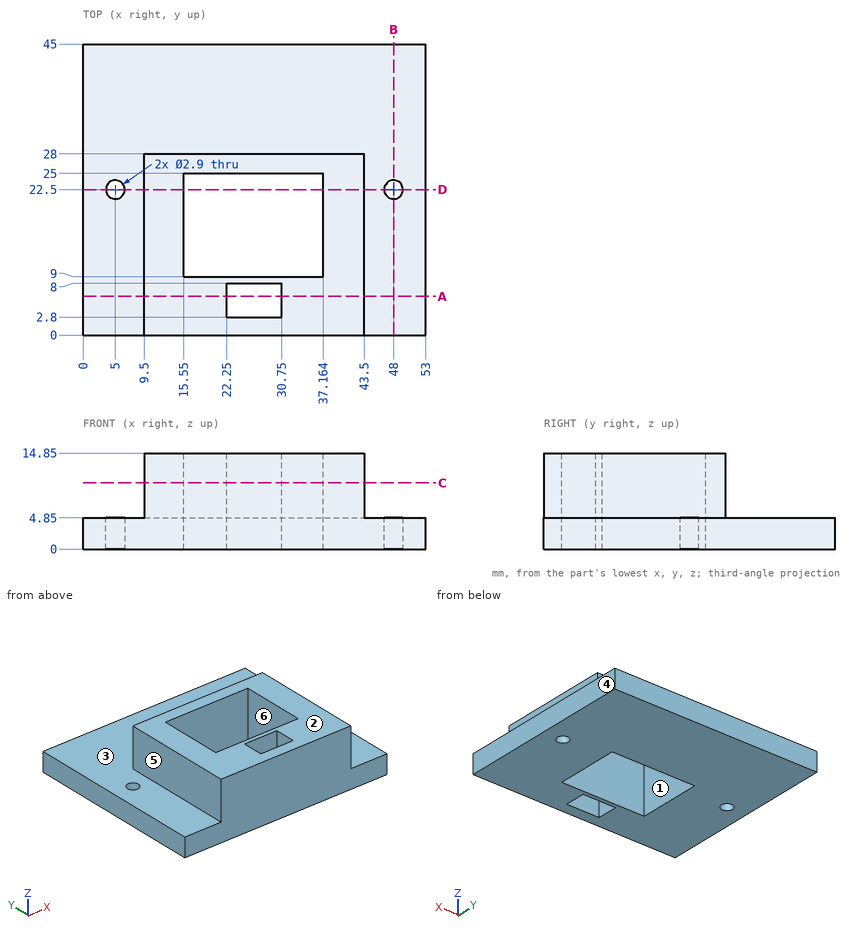
Design review of the part shown in the three views and the two pictorial views. Dimensions are in mm from the part's minimum x, y and z. A direction names the side the tool comes from. Round coordinates to 2 decimals unless told otherwise and drop trailing zeros. Loops run counter-clockwise (first coordinate to the right, second up) from the corner with the lowest first, then second, coordinate; pieces in that order, holes last. Notation, with made-up numbers: (40.25, 77) -> (80.25, 77) arc R19 ccw to (80.25, 83) -> close; hole circle Ø2 at (-2.75, 31.25). An arc over 180 degrees is marked (long way). Return JSON: item names as keys, results as strings.
(1) Add section C-C on z = 10.25. Write out the cut boundary in (x, y), plus the area to 3 significant figures.
Solved:
{"outline": "(9.5, 0) -> (43.5, 0) -> (43.5, 28) -> (9.5, 28) -> close; hole (15.55, 9) -> (37.16, 9) -> (37.16, 25) -> (15.55, 25) -> close; hole (22.25, 2.8) -> (30.75, 2.8) -> (30.75, 8) -> (22.25, 8) -> close", "area": "562 mm2"}
(2) Add section D-D on y = 22.5. Write out the cut boundary in (x, z).
Solved:
{"outline": "(0, 0) -> (3.55, 0) -> (3.55, 4.85) -> (0, 4.85) -> close; (6.45, 0) -> (15.55, 0) -> (15.55, 14.85) -> (9.5, 14.85) -> (9.5, 4.85) -> (6.45, 4.85) -> close; (37.16, 0) -> (46.55, 0) -> (46.55, 4.85) -> (43.5, 4.85) -> (43.5, 14.85) -> (37.16, 14.85) -> close; (49.45, 0) -> (53, 0) -> (53, 4.85) -> (49.45, 4.85) -> close"}
(3) Add section B-B on x = 48. Write out the cut boundary in (y, z), plus the area to 3 significant figures.
Solved:
{"outline": "(0, 0) -> (21.05, 0) -> (21.05, 4.85) -> (0, 4.85) -> close; (23.95, 0) -> (45, 0) -> (45, 4.85) -> (23.95, 4.85) -> close", "area": "204 mm2"}
(4) For line 1 (Y direction, x = 23, z = 4); line 2 (Y direction, x = 30.5, z = 10.25); line 3 (Y direction, x = 48, z = 1.75), list the stretches that pass through material, from the lowest coordinate up.
Solved:
{"line 1": "0 to 2.8, 8 to 9, 25 to 45", "line 2": "0 to 2.8, 8 to 9, 25 to 28", "line 3": "0 to 21.05, 23.95 to 45"}
(5) For pin 1 (3 mm diameter, centred on y = 17.5, z = 8.5, fed in from -X); pin 2 (2.5 mm diameter, centred on x = 5, y = 22.5, fed in from -Z); pin 3 (3 mm diameter, centred on x = 9, z = 6.5, fed in from +Y), all flat-tipped, find the tip position at first contact; note any pin that passes through.
Solved:
{"pin 1": "x = 9.5", "pin 2": "through", "pin 3": "y = 28"}
(6) The part is to be moulded in two halves that separate along X. For the marked faces 3, 4, 5 and 6, say which applies: released by +X, released by -X, zero draft, split by the parting line, or undercut.
Solved:
{"face 3": "zero draft", "face 4": "released by +X", "face 5": "released by -X", "face 6": "undercut"}
(7) For the marked faces 1 and 2, list the 3-axis set-ups (+Z, -Z, +X, -X, +Y, -Y) from which the entire face can be reached by the end or side of a thin tool; tool diameter is ignored.
Solved:
{"face 1": "+Z, -Z", "face 2": "+Z, +X, -X, +Y, -Y"}
(8) Add section A-A on y = 6. Write out the cut boundary in (x, z).
Solved:
{"outline": "(0, 0) -> (22.25, 0) -> (22.25, 14.85) -> (9.5, 14.85) -> (9.5, 4.85) -> (0, 4.85) -> close; (30.75, 0) -> (53, 0) -> (53, 4.85) -> (43.5, 4.85) -> (43.5, 14.85) -> (30.75, 14.85) -> close"}
